Design review of the part built by this model. Coordinates are the model's own, in mm. A direction names the side the tool comes from. Coordinates: 2 decimals unless noted, no trailing zeros. Write each loop counter-clockwise with the first axis right and the second up, starting at its lowest first coordinate (ties: lowest second). Pieces come first, ordered by that corner, then holes.
Q1. To check wall thickness, follow probe 1 along Y at (x, z) = (0.25, 40.5); probe 2 along Y at (x, z) = (0, 42) (3 decimals); probe 3 along X at (y, z) = (-0.5, 9.5). State the ranges of each line that lie inside material, in increasing order.
Q2. Clearance check with flat-ended pins moving along their axes: pin 1 Ø1 at (x, y) = (1, -2) entering from +Z; pin 2 Ø3 at (x, y) = (-3.5, 0) entering from -Z; pin 3 Ø1.5 at (y, z) = (3.5, 5.5) entering from +X. State where each tip first meets the part, or that it passes through.
Q3. Add section A-A, the plane z = 65. Give the boundary of the cut face in (x, y) (3 decimals).
Q4. Machinability: for faces 4 (the face through (0.59, -1.13, -28.27)), 5 (the face through (1.01, -1.01, -22.5)), which of the approach directions +Z, -Z, +X, -X, +Y, -Y give a long, thin tool a straight path to every point of the face, cutting with its end or side? Answer none if there is none.
Q5. The part is to be moulded in two halves that separate along Y. For faces 1 (the face through (-0.619, -2.787, 29.967)), 2 (the face through (1, -3, 80.5)), 3 (the face through (-4.292, 1.352, 26.288)), say which applies: +Y half, -Y half, draft (parallel to the pull), parting line (faces both ways), or undercut.
from build123d import *

# Parameters (mm, degrees)
F2_R     = 2.855
F3_DEPTH = 103
F4_R     = 1.275
F5_DEPTH = 25
F6_R     = 0.1
F7_SIZE  = 0.5
F8_R     = 5


with BuildPart() as f1:
    # F0 (on Front) → F1 (revolve)
    with BuildSketch(Plane.XZ):
        Polygon((-4.5, -27.5000141266), (0, -37.5000141266), (0, 80.4999858734), (-4.5, 80.4999858734), (-4.5, 45.166639983), align=None)
    revolve(axis=Axis((0, 0, 21.4999858734), (0, 0, -1)))

    # F2 (on face) → F3 (cut)
    with BuildSketch(Plane.XY.offset(80.4999858734)):
        Circle(F2_R)
    extrude(amount=-F3_DEPTH, mode=Mode.SUBTRACT)

    # F4 (on face) → F5 (cut)
    with BuildSketch(Plane.XY.offset(-22.5000141266)):
        Circle(F4_R)
    extrude(amount=-F5_DEPTH, mode=Mode.SUBTRACT)

    # F6
    f6_edges = [f1.edges().sort_by_distance(p)[0] for p in [
        (0, 1.275, -34.666681),
        (0, -1.275, -34.666681),
    ]]
    fillet(f6_edges, radius=F6_R)

    # F7
    f7_edges = [f1.edges().sort_by_distance(p)[0] for p in [
        (-2.855, 0, -22.500014),
    ]]
    chamfer(f7_edges, length=F7_SIZE)

    # F8
    f8_edges = [f1.edges().sort_by_distance(p)[0] for p in [
        (4.5, 0, -27.500014),
    ]]
    fillet(f8_edges, radius=F8_R)


solid = f1.part
Here are the results:
1. probe 1: y = -4.49 to -2.84, 2.84 to 4.49
1. probe 2: y = -4.5 to -2.855, 2.855 to 4.5
1. probe 3: x = -4.47 to -2.81, 2.81 to 4.47
2. pin 1: stops at z = -22.12
2. pin 2: stops at z = -33.06
2. pin 3: stops at x = 3.56
3. outline: circle Ø9 at (0, 0); hole circle Ø5.71 at (0, 0)
4. face 4: +Z, -Z
4. face 5: +Z
5. face 1: undercut
5. face 2: draft
5. face 3: parting line
